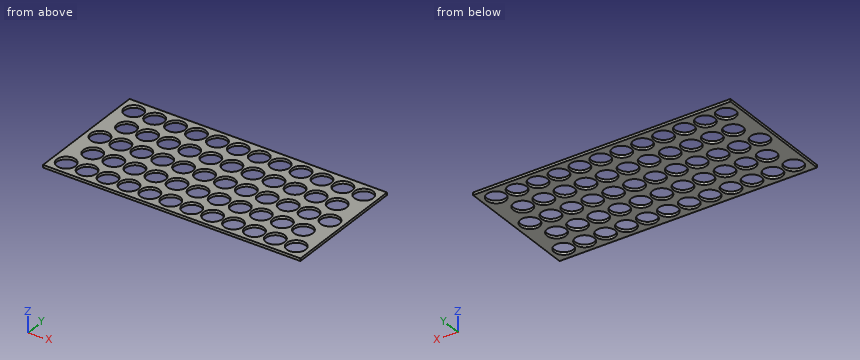
from build123d import *

# Parameters (mm, degrees)
F0_W     = 300
F0_H     = 146
F1_DEPTH = 3
F2_R     = 11
F3_DEPTH = 3.001


with BuildPart() as f1:
    # F0 (on Top) → F1 (new body)
    with BuildSketch(Plane.XY):
        with Locations((150, 73)):
            Rectangle(F0_W, F0_H)
    extrude(amount=F1_DEPTH)

    # F2 (on face) → F3 (cut, through all)
    with BuildSketch(Plane.XY.offset(3)):
        with Locations((16, 130)):
            Circle(F2_R)
        with Locations((40.363636, 130)):
            Circle(F2_R)
        with Locations((64.727273, 130)):
            Circle(F2_R)
        with Locations((89.090909, 130)):
            Circle(F2_R)
        with Locations((113.454545, 130)):
            Circle(F2_R)
        with Locations((137.818182, 130)):
            Circle(F2_R)
        with Locations((162.181818, 130)):
            Circle(F2_R)
        with Locations((186.545455, 130)):
            Circle(F2_R)
        with Locations((210.909091, 130)):
            Circle(F2_R)
        with Locations((235.272727, 130)):
            Circle(F2_R)
        with Locations((259.636364, 130)):
            Circle(F2_R)
        with Locations((284, 130)):
            Circle(F2_R)
        with Locations((16, 73)):
            Circle(F2_R)
        with Locations((40.363636, 73)):
            Circle(F2_R)
        with Locations((64.727273, 73)):
            Circle(F2_R)
        with Locations((89.090909, 73)):
            Circle(F2_R)
        with Locations((113.454545, 73)):
            Circle(F2_R)
        with Locations((137.818182, 73)):
            Circle(F2_R)
        with Locations((162.181818, 73)):
            Circle(F2_R)
        with Locations((186.545455, 73)):
            Circle(F2_R)
        with Locations((210.909091, 73)):
            Circle(F2_R)
        with Locations((235.272727, 73)):
            Circle(F2_R)
        with Locations((259.636364, 73)):
            Circle(F2_R)
        with Locations((284, 73)):
            Circle(F2_R)
        with Locations((16, 16)):
            Circle(F2_R)
        with Locations((40.363636, 16)):
            Circle(F2_R)
        with Locations((64.727273, 16)):
            Circle(F2_R)
        with Locations((89.090909, 16)):
            Circle(F2_R)
        with Locations((113.454545, 16)):
            Circle(F2_R)
        with Locations((137.818182, 16)):
            Circle(F2_R)
        with Locations((162.181818, 16)):
            Circle(F2_R)
        with Locations((186.545455, 16)):
            Circle(F2_R)
        with Locations((210.909091, 16)):
            Circle(F2_R)
        with Locations((235.272727, 16)):
            Circle(F2_R)
        with Locations((259.636364, 16)):
            Circle(F2_R)
        with Locations((284, 16)):
            Circle(F2_R)
        with Locations((27.3, 101.5)):
            Circle(F2_R)
        with Locations((27.3, 44.5)):
            Circle(F2_R)
        with Locations((51.84, 101.5)):
            Circle(F2_R)
        with Locations((51.84, 44.5)):
            Circle(F2_R)
        with Locations((76.38, 101.5)):
            Circle(F2_R)
        with Locations((76.38, 44.5)):
            Circle(F2_R)
        with Locations((100.92, 101.5)):
            Circle(F2_R)
        with Locations((100.92, 44.5)):
            Circle(F2_R)
        with Locations((125.46, 101.5)):
            Circle(F2_R)
        with Locations((125.46, 44.5)):
            Circle(F2_R)
        with Locations((150, 101.5)):
            Circle(F2_R)
        with Locations((150, 44.5)):
            Circle(F2_R)
        with Locations((174.54, 101.5)):
            Circle(F2_R)
        with Locations((174.54, 44.5)):
            Circle(F2_R)
        with Locations((199.08, 101.5)):
            Circle(F2_R)
        with Locations((199.08, 44.5)):
            Circle(F2_R)
        with Locations((223.62, 101.5)):
            Circle(F2_R)
        with Locations((223.62, 44.5)):
            Circle(F2_R)
        with Locations((248.16, 101.5)):
            Circle(F2_R)
        with Locations((248.16, 44.5)):
            Circle(F2_R)
        with Locations((272.7, 101.5)):
            Circle(F2_R)
        with Locations((272.7, 44.5)):
            Circle(F2_R)
    extrude(amount=-F3_DEPTH, mode=Mode.SUBTRACT)


solid = f1.part
Input: part model. Units: mm. Frame: model coordinates. Give positions to 0.01 mm unless a question says otherwise; leave off trailing zeros. Write each loop counter-clockwise with the first axis right and the second up, starting at its lowest first coordinate (ties: lowest second). Pieces come first, ordered by that corner, then holes.
Q1. Section A-A, the plane y = 101.5. State how many separate pieces and enclosed holes the cut face has, plus the area to 3 significant figures.
Q2. Section B-B, the plane x = 19. Output: boundary loops of the cut face in (y, z).
Q3. Material intervals for probe 1 along Y at (x, z) = (175.5, 2.5); probe 2 along Y at (x, z) = (162, 1.45); probe 3 along Y at (x, z) = (146.5, 2.15), sorted ascending.
Q4. First-contact query: P1, Ø3, axis at x = 182.5, y = 33, coming from the -Z side; P2, Ø17.5, axis at x = 174.54, y = 44.5, coming from the -Z side. Flat tips, straight axial feed; report the tip coordinate or a pass-through.
Filled in:
1. separate pieces: 12
1. enclosed holes: 0
1. area: 174 mm2
2. outline: (0, 0) - (5.42, 0) - (5.42, 3) - (0, 3) - close; (26.58, 0) - (37.28, 0) - (37.28, 3) - (26.58, 3) - close; (51.72, 0) - (62.42, 0) - (62.42, 3) - (51.72, 3) - close; (83.58, 0) - (94.28, 0) - (94.28, 3) - (83.58, 3) - close; (108.72, 0) - (119.42, 0) - (119.42, 3) - (108.72, 3) - close; (140.58, 0) - (146, 0) - (146, 3) - (140.58, 3) - close
3. probe 1: y = 0 to 33.54, 55.46 to 90.54, 112.46 to 146
3. probe 2: y = 0 to 5, 27 to 62, 84 to 119, 141 to 146
3. probe 3: y = 0 to 9.25, 22.75 to 34.07, 54.93 to 66.25, 79.75 to 91.07, 111.93 to 123.25, 136.75 to 146
4. P1: stops at z = 0
4. P2: passes through
